For this review, take the finished solid that the model builds, in its own axes (mm). A direction names the side the tool comes from. Round coordinates to 2 decimals unless told otherwise and drop trailing zeros. Order: outer loops, then holes, each group sorted by start corner. A loop starts at its lowest first (then second) coordinate and runs counter-clockwise, first axis right, second up. Notation, with made-up numbers: M 8,54.25 L 16,54.25 A24 ccw 16,72.25 Z; hole C -37.5,26.5 d1. An arc over 180 degrees is marked long. Put each result on its own line as item: value.
Autodesk Inventor part; units mm, degrees
ref_plane "YZ Plane" through (0, 0, 0) normal (1, 0, 0) x (0, 1, 0)
ref_plane "XZ Plane" through (0, 0, 0) normal (0, 1, 0) x (-1, 0, 0)
ref_plane "XY Plane" through (0, 0, 0) normal (0, 0, 1) x (1, 0, 0)
sketch "Sketch1" plane through (0, 0, 0) normal (0, 0, 1) x (1, 0, 0)
  circle A0 centre (54.61, 0) radius 7.395
  circle A1 centre (54.61, 0) radius 9.795
  point P0 (0, 0)
  dimension "d0" = 2.4
extrude "Extrusion1" add sketch "Sketch1" against normal blind 20
sketch "Sketch2" plane through (54.61, 0, 0) normal (0, 0, 1) x (1, 0, 0)
  circle A0 centre (0, 0) radius 7.395
  circle A1 centre (0, 0) radius 9.795
  circle A2 centre (0, 0) radius 2
  point P0 (-54.61, 0)
extrude "Extrusion2" add sketch "Sketch2" against normal blind 3 contours A0 | A1 | A2
sketch "Sketch3" plane through (54.61, 0, 0) normal (0, 0, 1) x (1, 0, 0)
  circle A0 centre (0, 0) radius 2
  point P0 (-54.61, 0)
extrude "Extrusion3" add sketch "Sketch3" along normal blind 15
chamfer "Chamfer1" distance 2 angle 45 1 edges at (52.61, 0, 0)
chamfer "Chamfer2" distance 0.6 angle 45 1 edges at (52.61, 0, 15)
chamfer "Chamfer3" distance 7.39 angle 45 1 edges at (47.215, 0, -3)
properties part number "Transmission_Mount_Tester"
(1) Add section D-D on z = -8. Give the boundary of the cut face in (x, y) (3 decimals).
A:
outline: C 54.61,0 d19.59; hole C 54.61,0 d10.01
(2) Add section B-B on y = 8. Give the boundary of the cut face in (x, z).
A:
outline: M 48.96,-20 L 60.26,-20 L 60.26,0 L 48.96,0 Z
(3) To check wall thickness, follow L1, parallel to Y at x = 54.61, z = -16.75 (3 decimals); L2, parallel to Z at x = 47.5, y = -5; L3, parallel to Y at x = 60, z = -17.5. State the ranges of each line that lie inside material, in increasing order.
A:
L1: y = -9.795 to -7.395, 7.395 to 9.795
L2: z = -20 to 0
L3: y = -8.18 to -5.06, 5.06 to 8.18
(4) Insertion check: pin 1 Ø2 at (y, z) = (-7, -5.5) entering from -X; pin 2 Ø5 at (x, z) = (51, 2) entering from -Y; pin 3 Ø5 at (x, y) = (50.5, -1) entering from -Z. Each pin has a flat end and moves straight along its axis. Give the tip position at first contact, or say it passes through.
A:
pin 1: stops at x = 46.87
pin 2: stops at y = -9.57
pin 3: stops at z = -9.72
(5) Draft analysis for pull direction Y (two halves, no side actions). For faces 1 (the face through (56.573, 0.814, 1.875)), 2 (the face through (47.222, 0.325, -15.128)), 3 (the face through (51, 7, -20)), state which applies: released by +Y, released by -Y, zero draft, split by the parting line, or undercut.
A:
face 1: split by the parting line
face 2: undercut
face 3: zero draft
(6) For faces 4 (the face through (55, 0, 15)), 5 (the face through (54.5, -4.2, 0)), list the 3-axis set-ups (+Z, -Z, +X, -X, +Y, -Y) from which the entire face can be reached by the end or side of a thin tool; tool diameter is ignored.
A:
face 4: +Z, +X, -X, +Y, -Y
face 5: +Z
(7) Add section A-A on z = 11. Give the boundary of the cut face in (x, y).
A:
outline: C 54.61,0 d4
(8) Add section C-C on x = 63. Give the boundary of the cut face in (y, z), then the cut area to 3 significant figures.
A:
outline: M -5.05,-20 L 5.05,-20 L 5.05,0 L -5.05,0 Z
area: 202 mm2
